```python
from build123d import *

# Parameters (mm, degrees)
ESQUISSE1_W                                    = 32
ESQUISSE1_H                                    = 18
BOSS_EXTRU_1_DEPTH                             = 2
ESQUISSE2_W                                    = 19
ESQUISSE2_H                                    = 14
BOSS_EXTRU_2_DEPTH                             = 1.4
FRAISAGE_POUR_VIS_T_TE_FRAIS_E_M21_D           = 2.6
FRAISAGE_POUR_VIS_T_TE_FRAIS_E_M21_CSINK_D     = 4.4
FRAISAGE_POUR_VIS_T_TE_FRAIS_E_M21_CSINK_ANGLE = 90
ESQUISSE6_W                                    = 15.8
ESQUISSE6_H                                    = 2
BOSS_EXTRU_3_DEPTH                             = 18
ESQUISSE7_W                                    = 19.2
ESQUISSE7_H                                    = 1.2
BOSS_EXTRU_4_DEPTH                             = 21
CONG_5_R                                       = 1


with BuildPart() as part:
    # Esquisse1 → Boss.-Extru.1 (new body)
    with BuildSketch(Plane.XY):
        Rectangle(ESQUISSE1_W, ESQUISSE1_H)
    extrude(amount=BOSS_EXTRU_1_DEPTH)

    # Esquisse2 → Boss.-Extru.2 (add)
    with BuildSketch(Plane(origin=(0, 0, 0), x_dir=(-1, 0, 0), z_dir=(0, 0, -1))):
        Rectangle(ESQUISSE2_W, ESQUISSE2_H)
    extrude(amount=BOSS_EXTRU_2_DEPTH)

    # Fraisage pour vis à tête fraisée M21 (through all)
    with Locations(Plane.XY.offset(2)):
        with Locations((-13, 0)):
            fraisage_pour_vis_t_te_frais_e_m21 = CounterSinkHole(FRAISAGE_POUR_VIS_T_TE_FRAIS_E_M21_D / 2, FRAISAGE_POUR_VIS_T_TE_FRAIS_E_M21_CSINK_D / 2, counter_sink_angle=FRAISAGE_POUR_VIS_T_TE_FRAIS_E_M21_CSINK_ANGLE)

    # Symétrie1: Fraisage pour vis à tête fraisée M21 across plane
    add(fraisage_pour_vis_t_te_frais_e_m21.mirror(Plane(origin=(0, 0, 0), x_dir=(0, 0, 1), z_dir=(1, 0, 0))), mode=Mode.SUBTRACT)

    # Esquisse6 → Boss.-Extru.3 (add)
    with BuildSketch(Plane(origin=(0, 0, 0), x_dir=(-1, 0, 0), z_dir=(0, 0, -1))):
        with Locations((0, 8)):
            Rectangle(ESQUISSE6_W, ESQUISSE6_H)
    extrude(amount=BOSS_EXTRU_3_DEPTH)

    # Esquisse7 → Boss.-Extru.4 (add)
    with BuildSketch(Plane.XY.offset(2)):
        with Locations((0, 6.4)):
            Rectangle(ESQUISSE7_W, ESQUISSE7_H)
    extrude(amount=-BOSS_EXTRU_4_DEPTH)

    # Congé5
    cong_5_edges = [part.edges().sort_by_distance(p)[0] for p in [
        (9.6, 6.4, -19),
        (-9.6, 6.4, -19),
        (16, -9, 1),
        (-16, -9, 1),
    ]]
    fillet(cong_5_edges, radius=CONG_5_R)


solid = part.part
```
Part model, mm, in its own coordinate system. A direction names the side the tool comes from. Coordinates: 2 decimals unless noted, no trailing zeros. Write each loop counter-clockwise with the first axis right and the second up, starting at its lowest first coordinate (ties: lowest second). Pieces come first, ordered by that corner, then holes.
Item 1: Probe line 1 (X direction, y = 0, z = 0.7); line 2 (Y direction, x = -13, z = 0.3); line 3 (Z direction, x = -6, y = -3.5). List the from-to ranges inside material, lowest first.
Item 2: Slice it at C-C (z = -9.5). Write the cut outline in (x, y).
Item 3: Pin check, flat tips, straight feed: pin 1 (1 mm diameter, centred on y = 8, z = -9.5, fed in from +X); pin 2 (1.1 mm diameter, centred on x = 0.5, z = -1, fed in from -Y); pin 3 (0.6 mm diameter, centred on x = 0.5, y = 8, fed in from -Z); pin 4 (8 mm diameter, centred on y = -0.5, z = -12, fed in from -X). Stop position of each tip, or through.
Item 4: Slice it at B-B (y = 0). Write the cut outline in (x, z).
Item 5: Mould opens along X. For faces 4 (the face through (-15.699, -8.715, 1.014)), 5 (the face through (9.5, -1, -1)), 6 (the face through (-14.24, 0.39, 0.54)) say: released by +X, released by -X, zero draft, split by the parting line, or undercut.
Item 6: Slice it at A-A (x = 13). Write the cut outline in (y, z), and give its area (3 significant figures).
Item 7: Which spindle directions (+Z, -Z, +X, -X, +Y, -Y) get a long thin tool onto all of the face, cutting with end or side? Do faces 1 (the face through (-9.5, -1, -1)), 2 (the face through (0, 8, -18)), 3 (the face through (-7.9, 8, -9)). Say none if no direction does.
Item 8: Slice it at D-D (x = 1). Write the cut outline in (y, z), and give its area (3 significant figures).
Results found:
1. line 1: x = -16 to -14.3, -11.7 to 11.7, 14.3 to 16
1. line 2: y = -9 to -1.3, 1.3 to 9
1. line 3: z = -1.4 to 2
2. outline: (-9.6, 5.8) - (9.6, 5.8) - (9.6, 7) - (7.9, 7) - (7.9, 9) - (-7.9, 9) - (-7.9, 7) - (-9.6, 7) - close
3. pin 1: stops at x = 7.9
3. pin 2: stops at y = -7
3. pin 3: stops at z = -18
3. pin 4: passes through
4. outline: (-16, 0) - (-14.3, 0) - (-14.3, 1.1) - (-15.2, 2) - (-16, 2) - close; (-11.7, 0) - (-9.5, 0) - (-9.5, -1.4) - (9.5, -1.4) - (9.5, 0) - (11.7, 0) - (11.7, 1.1) - (10.8, 2) - (-10.8, 2) - (-11.7, 1.1) - close; (14.3, 0) - (16, 0) - (16, 2) - (15.2, 2) - (14.3, 1.1) - close
5. face 4: released by -X
5. face 5: released by +X
5. face 6: undercut
6. outline: (-9, 0) - (-1.3, 0) - (-1.3, 1.1) - (-2.2, 2) - (-9, 2) - close; (1.3, 0) - (9, 0) - (9, 2) - (2.2, 2) - (1.3, 1.1) - close
6. area: 30.0 mm2
7. face 1: -Z, -X, -Y
7. face 2: -Z, +X, -X, +Y
7. face 3: -Z, -X, +Y
8. outline: (-9, 0) - (-7, 0) - (-7, -1.4) - (5.8, -1.4) - (5.8, -19) - (7, -19) - (7, -18) - (9, -18) - (9, 2) - (-9, 2) - close
8. area: 113 mm2
